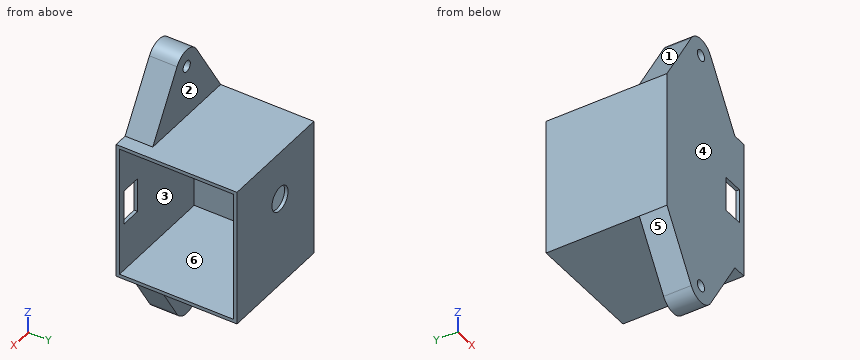
Autodesk Inventor part; units mm, degrees
ref_plane "YZ Plane" through (0, 0, 0) normal (1, 0, 0) x (0, 1, 0)
ref_plane "XZ Plane" through (0, 0, 0) normal (0, 1, 0) x (-1, 0, 0)
ref_plane "XY Plane" through (0, 0, 0) normal (0, 0, 1) x (1, 0, 0)
sketch "Sketch1" plane through (0, 0, 0) normal (0, 1, 0) x (-1, 0, 0)
  line L0 (-15, 20) -> (15, 20)
  line L1 (15, 20) -> (15, -20)
  line L2 (15, -20) -> (-15, -20)
  line L3 (-15, -20) -> (-15, 20)
  line L4 (-15, 20) -> (15, -20) construction
  line L5 (15, 20) -> (-15, -20) construction
  line L6 (0, 31.25) -> (0, -31.25)
  point P0 (0, 0)
  dimension "d0" = 30
  dimension "d1" = 40
  dimension "d2" = 62.5
  dimension "d3" = 18.75
extrude "Extrusion1" add sketch "Sketch1" along normal blind 35
shell "Shell1" thickness 1 removed faces 1 at (15, 11.6667, 6.6667)
sketch "Sketch3" plane through (0, 35, 0) normal (0, 1, 0) x (1, 0, 0)
  point P0 (0, 0)
sketch "Sketch4" plane through (0, 0, 0) normal (0, 1, 0) x (-1, 0, 0)
  arc A0 (-4.2693, -37.6026) -> (4.2693, -37.6026) centre (0, -35) ccw
  line L0 (-15, -20) -> (15, -20)
  line L1 (28.6058, 0) -> (-27.8274, 0)
  line L2 (15, -20) -> (15, 20)
  arc A1 (4.2693, 37.6026) -> (-4.2693, 37.6026) centre (0, 35) ccw
  line L3 (15, -20) -> (4.2693, -37.6026)
  line L4 (-15, -20) -> (-4.2693, -37.6026)
  line L5 (15, 20) -> (-15, 20)
  line L6 (-15, 20) -> (-4.2693, 37.6026)
  line L7 (15, 20) -> (4.2693, 37.6026)
  circle A2 centre (0, -35) radius 1.6
  circle A3 centre (0, 35) radius 1.6
  point P0 (0, 0)
  point P1 (0, -20)
  point P2 (0.3892, 0)
  point P3 (15, 0)
  dimension "d7" = 10
  dimension "d8" = 15
  dimension "d9" = 3.2
  dimension "d10" = 3.2
extrude "Extrusion2" add sketch "Sketch4" along normal blind 8
sketch "Sketch5" plane through (0, 35, 0) normal (0, 1, 0) x (1, 0, 0)
  circle A0 centre (0, -6) radius 3.55
  point P0 (0, 0)
  dimension "d15" = 7.1
  dimension "d16" = 6
extrude "Extrusion3" cut sketch "Sketch5" against normal blind 10
sketch "Sketch6" plane through (15, 0, 20) normal (1, 0, 0) x (0, 0, -1)
  point P0 (20, 0)
sketch "Sketch7" plane through (15, 35, 20) normal (1, 0, 0) x (0, 0, -1)
  line L0 (0, -27) -> (0, 0)
  line L1 (40, -35) -> (0, -35)
  line L2 (0, -35) -> (0, 0)
  line L3 (0, 0) -> (40, 0)
  line L4 (40, 0) -> (40, -35)
  line L5 (40, -35) -> (0, 0) construction
  line L6 (0, -35) -> (40, 0) construction
  line L7 (1, -34) -> (1, -1)
  line L8 (0, 0) -> (40, 0)
  line L9 (1, -1) -> (39, -1)
  line L10 (1, -34) -> (39, -34)
  line L11 (39, -34) -> (39, -1)
  line L12 (39, -1) -> (1, -1)
  line L13 (1, -1) -> (1, -34)
  line L14 (1, -34) -> (39, -1) construction
  line L15 (39, -34) -> (1, -1) construction
  point P0 (20, -35)
  point P1 (0, -25)
  point P2 (20, -17.5)
  point P3 (20, 0)
  point P4 (1, -17.5)
  point P5 (0, -17.5)
  point P6 (20, -35)
  point P7 (20, 0)
  point P8 (0, -25)
extrude "Extrusion4" add sketch "Sketch7" along normal blind 4
sketch "Sketch9" plane through (-14, 1, 19) normal (0, 1, 0) x (1, 0, 0)
  line L0 (25, 24) -> (31, 24)
  line L1 (31, 24) -> (31, 14)
  line L2 (31, 14) -> (25, 14)
  line L3 (25, 14) -> (25, 24)
  line L4 (25, 24) -> (31, 14) construction
  line L5 (31, 24) -> (25, 14) construction
  line L6 (33, 38) -> (33, 0)
  point P0 (14, 19)
  point P1 (28, 19)
  point P2 (33, 19)
  point P3 (33, 19)
  dimension "d25" = 6
  dimension "d26" = 10
  dimension "d27" = 5
extrude "Extrusion6" cut sketch "Sketch9" against normal through all
properties part number "SERVO BASE HOUSING_3DPrint"
Read the model definition and answer for the solid it produces. Units are mm, in the model's axes. Face numbers are marked on the shaded views. A direction names the side the tool comes from. Round coordinates to 2 decimals unless told otherwise and drop trailing zeros. Order: outer loops, then holes, each group sorted by start corner. A loop starts at its lowest first (then second) coordinate and runs counter-clockwise, first axis right, second up.
1) The part is cut by section D-D on z = -6.5. Write down the section's boundary in (x, y), plus the area to 3 significant figures.
2) For the marked faces 1, 2 and 3, determine the directions among +Z, -Z, +X, -X, +Y, -Y from which every point of the face is accessible in a straight line to the end or side of a thin tool.
3) Straight lines are drawn through the part: L1, parallel to Z at x = 0, y = 3; L2, parallel to Z at x = -8, y = 21; L3, parallel to Y at x = 10, z = -6. For each, find the intervals that lie inside material, in ascending order.
4) The part is cut by section B-B on x = 0. Write down the section's boundary in (y, z), plus the area to 3 significant figures.
5) The mould has two halves that part along Y. Classify the marked faces 4, 5 and 6: released by +Y, released by -Y, zero draft, split by the parting line, or undercut.
6) The part is cut by section A-A on z = 6. Write down the section's boundary in (x, y), plus the area to 3 significant figures.
7) The part is cut by section C-C on y = 13.5. Write down the section's boundary in (x, z).
8) Flat-ended cylindrical pins translate along their axes: pin 1 (0.5 mm diameter, centred on x = 14, y = 0.5, fed in from +Z); pin 2 (16.5 mm diameter, centred on x = -3, y = 21, fed in from -Z); pin 3 (10 mm diameter, centred on x = -2, z = 26.5, fed in from +Y). Find the tip coordinate at first contact, or state that the pin passes through.
Resolved:
1. outline: (-15, 0) - (19, 0) - (19, 1) - (-14, 1) - (-14, 34) - (19, 34) - (19, 35) - (-15, 35) - close
1. area: 101 mm2
2. face 1: +Z, -X, +Y, -Y
2. face 2: +Z, +X, -X, +Y
2. face 3: +X
3. L1: z = -40 to -36.6, -33.4 to -19, 19 to 33.4, 36.6 to 40
3. L2: z = -20 to -19, 19 to 20
3. L3: y = 0 to 1, 34 to 35
4. outline: (0, -40) - (8, -40) - (8, -36.6) - (0, -36.6) - close; (0, -33.4) - (8, -33.4) - (8, -20) - (35, -20) - (35, 2.45) - (34, 2.45) - (34, -19) - (1, -19) - (1, 19) - (34, 19) - (34, 9.55) - (35, 9.55) - (35, 20) - (8, 20) - (8, 33.4) - (0, 33.4) - close; (0, 36.6) - (8, 36.6) - (8, 40) - (0, 40) - close
4. area: 408 mm2
5. face 4: released by -Y
5. face 5: zero draft
5. face 6: undercut
6. outline: (-15, 0) - (19, 0) - (19, 1) - (-14, 1) - (-14, 34) - (-3.55, 34) - (-3.55, 35) - (-15, 35) - close; (3.55, 34) - (19, 34) - (19, 35) - (3.55, 35) - close
6. area: 93.9 mm2
7. outline: (-15, -20) - (19, -20) - (19, -19) - (-14, -19) - (-14, 19) - (19, 19) - (19, 20) - (-15, 20) - close
8. pin 1: stops at z = 22.05
8. pin 2: stops at z = -20
8. pin 3: stops at y = 8
